```python
from build123d import *

# Parameters (mm, degrees)
F1_DEPTH = 228.6


with BuildPart() as f1:
    # F0 (on Right) → F1 (new body)
    with BuildSketch(Plane.YZ):
        with BuildLine():
            Line((4.490128, 4.490128), (0, 0))
            Line((0, 0), (33.67596, -33.67596))
            ThreePointArc((33.67596, -33.67596), (35.921024, -34.605896), (38.166089, -33.67596))
            ThreePointArc((38.166089, -33.67596), (39.096024, -31.430896), (38.166089, -29.185832))
            Line((38.166089, -29.185832), (4.490128, 4.490128))
        make_face()
    extrude(amount=-F1_DEPTH)


solid = f1.part
```
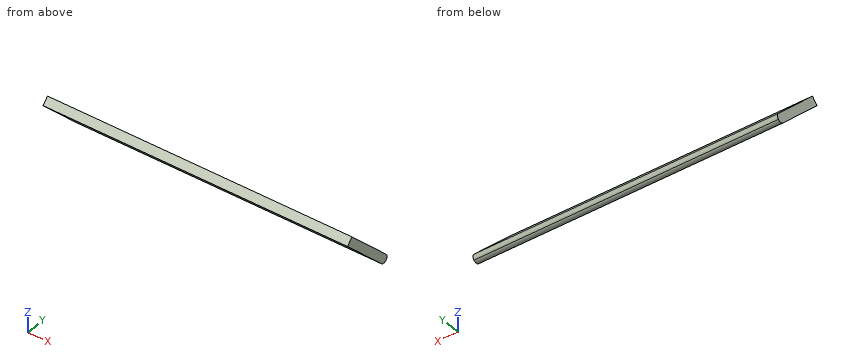
The model under review builds one solid part; all positions refer to its coordinate system, in mm. Give positions to 0.01 mm unless a question says otherwise; leave off trailing zeros. Write each loop counter-clockwise with the first axis right and the second up, starting at its lowest first coordinate (ties: lowest second). Pieces come first, ordered by that corner, then holes. Notation, with made-up numbers: (10, 8.5) -> (48, 8.5) arc R26 cw to (48, 41.5) -> close; hole circle Ø1 at (19, 0). An arc over 180 degrees is marked (long way). Answer in a Markdown table with one row per item.
1) Add section B-B on z = -3.5. State the section outline as (x, y) points.
Worked answers:
| item | result |
|---|---|
| outline | (-228.6, 3.5) -> (0, 3.5) -> (0, 12.48) -> (-228.6, 12.48) -> close |
2) Add section A-A on x = -92.5. State the section outline as (y, z) points (3 decimals), plus the area to 3 significant figures.
Worked answers:
| item | result |
|---|---|
| outline | (0, 0) -> (33.676, -33.676) arc R3.175 ccw to (38.166, -33.676) arc R3.175 ccw to (38.166, -29.186) -> (4.49, 4.49) -> close |
| area | 318 mm² |
3) For L1, parallel to Z at x = -29, y = 27; L2, parallel to Z at x = -186, y = 28; L3, parallel to Y at x = -217, z = -2.5, list the stretches that pass through material, from the lowest coordinate up. Write a range as [from, to].
Worked answers:
| item | result |
|---|---|
| L1 | [-27, -18.02] |
| L2 | [-28, -19.02] |
| L3 | [2.5, 11.48] |
4) Clearance check with flat-ended pins moving along their axes: P1, Ø1.5, axis at x = -113, z = -16.5, coming from the +Y side; P2, Ø1, axis at x = -100.5, z = -11, coming from the -Y side; P3, Ø6, axis at x = -62, z = -23, coming from the -Y side. State where each tip first meets the part, or that it passes through.
Worked answers:
| item | result |
|---|---|
| P1 | y = 26.23 |
| P2 | y = 10.5 |
| P3 | y = 20 |
5) Add section C-C on y = 8. State the section outline as (x, z) points, plus the area to 3 significant figures.
Worked answers:
| item | result |
|---|---|
| outline | (-228.6, -8) -> (0, -8) -> (0, 0.98) -> (-228.6, 0.98) -> close |
| area | 2,050 mm² |
